Can you work these out from the drawing? Everything is in mm from the part's minimum corner. A direction names the side the tool comes from. Coordinates: 2 decimals unless noted, no trailing zeros. Loops run counter-clockwise (first coordinate to the right, second up) from the corner with the lowest first, then second, coordinate; pieces in that order, holes last.
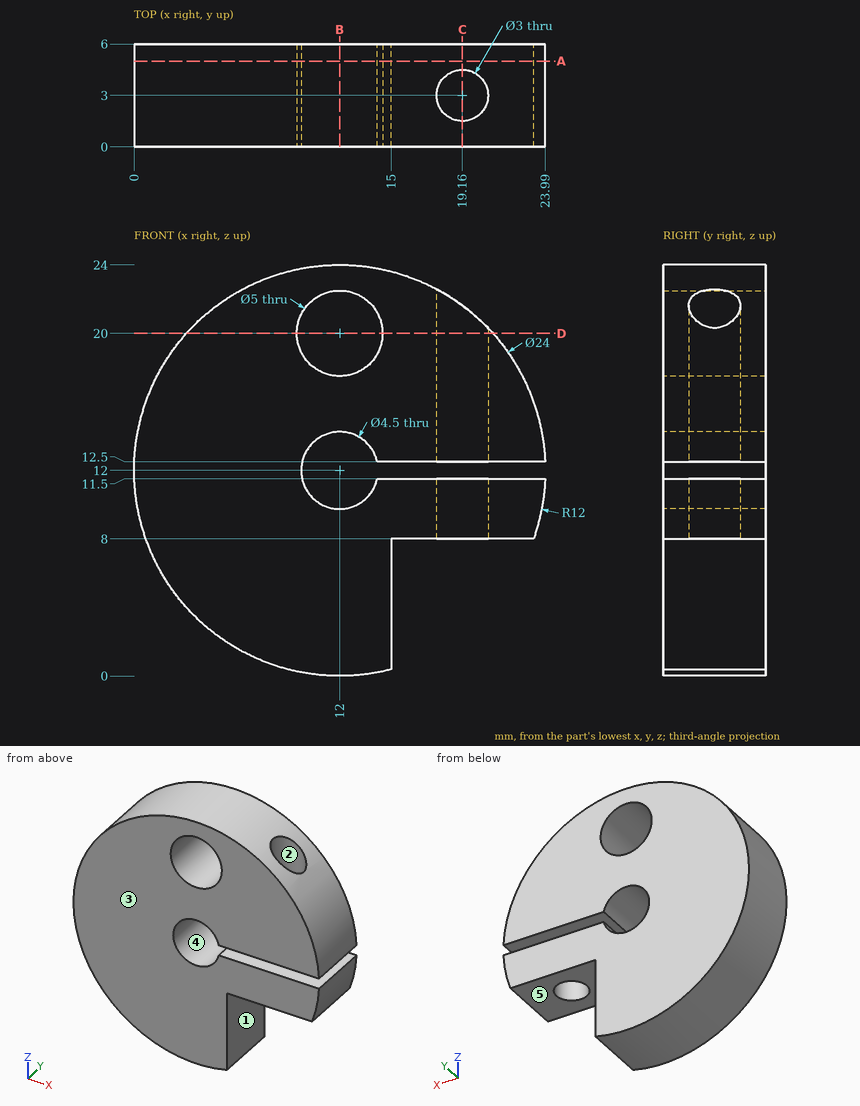
1. We'd pull the mould along Z, two halves only. Please class the marked faces 3, 4 and 5: +Z half, -Z half, draft (parallel to the pull), parting line (faces both ways), or undercut.
2. On a 3-axis mill with a long thin cutter (end or side, diameter ignored), from which of +Z, -Z, +X, -X, +Y, -Y can I reach the whole of each face in a straight line? I mean the marked faces 1 and 2. Say none if no direction works.
3. I want a section at C-C (x = 19.16). Please give me the cut outline in (y, z).
4. For pin 1 (6 mm diameter, centred on x = 12, z = 20, fed in from -Y); pin 2 (3 mm diameter, centred on x = 20.5, y = 5, fed in from +Z); pin 3 (1.5 mm diameter, centred on y = 3, z = 9.5, fed in from +X); pin 4 (1 mm diameter, centred on y = 4, z = 4.5, fed in from -X), each with a flat end and sliding along its axis, tell me the tip position at first contact or that it passes through.
5. I want a section at A-A (y = 5). Please give me the cut outline in (x, z).
6. I need wall thicknesses on line 1 along Y through (x, z) = (19.16, 20.25); line 2 along Z through (x, y) = (10.75, 0.5) (1 decimal); line 3 along X through (y, z) = (2, 10.5) (1 decimal). Which ranges of each line are inside material? Lowest first, please.
7. I want a section at D-D (z = 20). Please give me the cut outline in (x, y) (1 decimal).
8. I want a section at B-B (x = 12). Please give me the cut outline in (y, z).
Response values:
1. face 3: draft
1. face 4: undercut
1. face 5: -Z half
2. face 1: -Z, +X, +Y, -Y
2. face 2: +Z, -Z
3. outline: (0, 8) - (1.5, 8) - (1.5, 11.5) - (0, 11.5) - close; (0, 12.5) - (1.5, 12.5) - (1.5, 21.63) - (0, 21.63) - close; (4.5, 8) - (6, 8) - (6, 11.5) - (4.5, 11.5) - close; (4.5, 12.5) - (6, 12.5) - (6, 21.63) - (4.5, 21.63) - close
4. pin 1: stops at y = 0
4. pin 2: stops at z = 21.75
4. pin 3: stops at x = 23.87
4. pin 4: stops at x = 2.25
5. outline: (14.19, 11.5) arc R2.25 cw (long way) to (14.19, 12.5) - (23.99, 12.5) arc R12 ccw (long way) to (15, 0.38) - (15, 8) - (23.31, 8) arc R12 ccw to (23.99, 11.5) - close; hole circle Ø5 at (12, 20)
6. line 1: y = 0 to 1.5, 4.5 to 6
6. line 2: z = 0.1 to 10.1, 13.9 to 17.8, 22.2 to 23.9
6. line 3: x = 0.1 to 10.3, 13.7 to 18, 20.3 to 23.9
7. outline: (3.1, 0) - (9.5, 0) - (9.5, 6) - (3.1, 6) - close; (14.5, 0) - (20.9, 0) - (20.9, 6) - (14.5, 6) - close; hole circle Ø3 at (19.2, 3)
8. outline: (0, 0) - (6, 0) - (6, 9.75) - (0, 9.75) - close; (0, 14.25) - (6, 14.25) - (6, 17.5) - (0, 17.5) - close; (0, 22.5) - (6, 22.5) - (6, 24) - (0, 24) - close
